Read the model definition and answer for the solid it produces. Units are mm, in the model's axes. Face numbers are marked on the shaded views. A direction names the side the tool comes from. Coordinates: 2 decimals unless noted, no trailing zeros. Loops run counter-clockwise (first coordinate to the right, second up) from the corner with the lowest first, then second, coordinate; pieces in that order, holes last. Notation, with made-up numbers: (5, -8.5) -> (64, -8.5) arc R30 cw to (64, 17.5) -> close; hole circle Ø2 at (15, 63.5). An arc over 180 degrees is marked (long way). Answer in a Markdown table with one row per item.
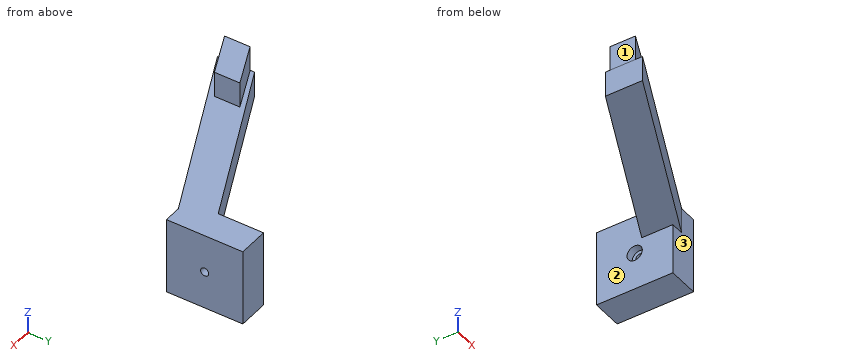
```python
from build123d import *

# Parameters (mm, degrees)
SKETCH_W        = 12
SKETCH_H        = 30
PAD_DEPTH       = 30
PAD001_DEPTH    = 10
SKETCH004_R     = 3
POCKET001_DEPTH = 3
SKETCH005_R     = 1.6
POCKET_DEPTH    = 9.001
PAD002_DEPTH    = 10


with BuildPart() as part:
    # Sketch → Pad (new body)
    with BuildSketch(Plane.XY):
        Rectangle(SKETCH_W, SKETCH_H)
    extrude(amount=PAD_DEPTH)

    # Sketch001 → Pad001 (join)
    with BuildSketch(Plane.XY.offset(30)):
        Polygon((0, 0), (-73.854295, -34.438823), (-73.854295, -49.021726), (0, -14.582903), align=None)
    extrude(amount=-PAD001_DEPTH)

    # Sketch004 → Pocket001 (cut)
    with BuildSketch(Plane.YZ.offset(-6)):
        with Locations((0, 14.871989)):
            Circle(SKETCH004_R)
    extrude(amount=POCKET001_DEPTH, mode=Mode.SUBTRACT)

    # Sketch005 → Pocket (cut, through all)
    with BuildSketch(Plane.YZ.offset(-3)):
        with Locations((0, 14.898449)):
            Circle(SKETCH005_R)
    extrude(amount=POCKET_DEPTH, mode=Mode.SUBTRACT)

    # Sketch006 → Pad002 (join)
    with BuildSketch(Plane.XY.offset(30)):
        Polygon((-73.59462, -36.062692), (-56.065701, -28.186142), (-56.065701, -38.186142), (-73.59462, -46.062692), align=None)
    extrude(amount=PAD002_DEPTH)


solid = part.part
```
1. A cutting plane is placed at C-C on x = -64. Give the vertices of the cut face in (y, z).
A:
| item | result |
|---|---|
| outline | (-44.43, 20) -> (-29.84, 20) -> (-29.84, 30) -> (-31.75, 30) -> (-31.75, 40) -> (-41.75, 40) -> (-41.75, 30) -> (-44.43, 30) -> close |
2. A tool of negligible diameter and unlimited length cuts with its end or side. For the marked faces 1, 2 and 3, from which of +Z, -Z, +X, -X, +Y, -Y can it reach the whole face along a straight path? Write none if from no direction.
A:
| item | result |
|---|---|
| face 1 | +Z, -X, +Y, -Y |
| face 2 | -Z, -X, +Y |
| face 3 | -Z, +X, -Y |
3. A cutting plane is placed at D-D on z = 6.5. Give the vertices of the cut face in (x, y), and give its area (3 significant figures).
A:
| item | result |
|---|---|
| outline | (-6, -15) -> (6, -15) -> (6, 15) -> (-6, 15) -> close |
| area | 360 mm2 |
4. A cutting plane is placed at A-A on y = 0. Give the vertices of the cut face in (x, z), and give its area (3 significant figures).
A:
| item | result |
|---|---|
| outline | (-6, 0) -> (6, 0) -> (6, 13.3) -> (-3, 13.3) -> (-3, 11.87) -> (-6, 11.87) -> close; (-6, 17.87) -> (-3, 17.87) -> (-3, 16.5) -> (6, 16.5) -> (6, 30) -> (-6, 30) -> close |
| area | 313 mm2 |
5. Find the intervals of material crossed by probe 1 along Z at (x, y) = (0, 0); probe 2 along Z at (x, y) = (-5, 0); probe 3 along X at (y, z) = (-1, 22), in increasing order.
A:
| item | result |
|---|---|
| probe 1 | z = 0 to 13.3, 16.5 to 30 |
| probe 2 | z = 0 to 11.87, 17.87 to 30 |
| probe 3 | x = -6 to 6 |
6. Given pin 1 Ø2 at (y, z) = (-8.5, 20) entering from -X; pin 2 Ø8 at (y, z) = (-39.5, 37.5) entering from -X; pin 3 Ø8 at (x, z) = (-12.5, 25) entering from +Y; pin 4 Ø3 at (y, z) = (0, 14.9) entering from -X, each flat-ended and moving along its own axis, determine where each tip first touches the part or whether it passes through.
A:
| item | result |
|---|---|
| pin 1 | stops at x = -20.37 |
| pin 2 | stops at x = -73.59 |
| pin 3 | stops at y = -3.96 |
| pin 4 | passes through |
7. A cutting plane is placed at B-B on z = 26. Give the vertices of the cut face in (x, y), and give its area (3 significant figures).
A:
| item | result |
|---|---|
| outline | (-73.85, -49.02) -> (-0.89, -15) -> (6, -15) -> (6, 15) -> (-6, 15) -> (-6, -2.8) -> (-73.85, -34.44) -> close |
| area | 1,360 mm2 |
